Check sheet for the modelled part. Datum: model origin and axes. Units: mm. Face numbers are marked on the shaded views. A direction names the side the tool comes from. Give positions to 0.01 mm unless a question says otherwise; leave off trailing zeros. Loops run counter-clockwise (first coordinate to the right, second up) from the corner with the lowest first, then second, coordinate; pieces in that order, holes last.
```python
from build123d import *

# Parameters (mm, degrees)
F0_W     = 100.33
F0_H     = 52.07
F1_DEPTH = 17.272
F2_R     = 5.08
F3_W     = 87.63
F3_H     = 39.37
F4_DEPTH = 25.4


with BuildPart() as f1:
    # F0 (on Top) → F1 (new body)
    with BuildSketch(Plane.XY):
        with Locations((50.165, 26.035)):
            Rectangle(F0_W, F0_H)
    extrude(amount=F1_DEPTH)

    # F2
    f2_edges = [f1.edges().sort_by_distance(p)[0] for p in [
        (0, 52.07, 8.636),
        (0, 0, 8.636),
        (100.33, 0, 8.636),
        (100.33, 52.07, 8.636),
    ]]
    fillet(f2_edges, radius=F2_R)

    # F3 (on face) → F4 (cut)
    with BuildSketch(Plane.XY.offset(17.272)):
        with Locations((50.165, 26.035)):
            Rectangle(F3_W, F3_H)
    extrude(amount=-F4_DEPTH, mode=Mode.SUBTRACT)


solid = f1.part
```
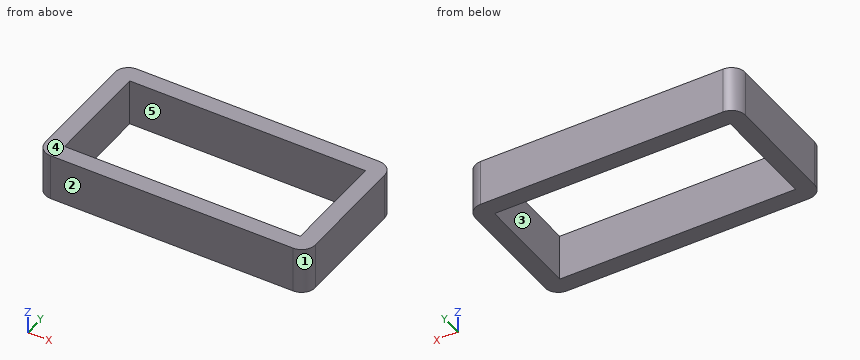
(1) Section check C-C on x = 21. Record the boundary of the cut face in (y, z), plus the area to 3 significant figures.
(2) Material ranges on line 1 (Y direction, x = 61, z = 5.75); line 2 (X direction, y = 25.5, z = 14.25); line 3 (Y direction, x = 95.5, z = 11.5), recorded low to high.
(3) Access from +Z, -Z, +X, -X, +Y, -Y to the whole of each face (thin tool, end or side, straight path). Record for the marked faces 4 and 5.
(4) Section check B-B on z = 2. Record the boundary of the cut face in (x, y).
(5) Release check for a two-part mould opening along X. For the marked faces 1, 2 and 3 record: pulls with the +X half, pulls with the -X half, needs draft (parallel to the pull), parting line crosses it, or undercut.
(6) Section check A-A on y = 37.5. Record the boundary of the cut face in (x, z).
Computed values:
1. outline: (0, 0) - (6.35, 0) - (6.35, 17.27) - (0, 17.27) - close; (45.72, 0) - (52.07, 0) - (52.07, 17.27) - (45.72, 17.27) - close
1. area: 219 mm2
2. line 1: y = 0 to 6.35, 45.72 to 52.07
2. line 2: x = 0 to 6.35, 93.98 to 100.33
2. line 3: y = 0.01 to 52.06
3. face 4: +Z, +X, -X, +Y, -Y
3. face 5: +Z, -Z
4. outline: (0, 5.08) arc R5.08 ccw to (5.08, 0) - (95.25, 0) arc R5.08 ccw to (100.33, 5.08) - (100.33, 46.99) arc R5.08 ccw to (95.25, 52.07) - (5.08, 52.07) arc R5.08 ccw to (0, 46.99) - close; hole (6.35, 6.35) - (93.98, 6.35) - (93.98, 45.72) - (6.35, 45.72) - close
5. face 1: pulls with the +X half
5. face 2: needs draft
5. face 3: undercut
6. outline: (0, 0) - (6.35, 0) - (6.35, 17.27) - (0, 17.27) - close; (93.98, 0) - (100.33, 0) - (100.33, 17.27) - (93.98, 17.27) - close
